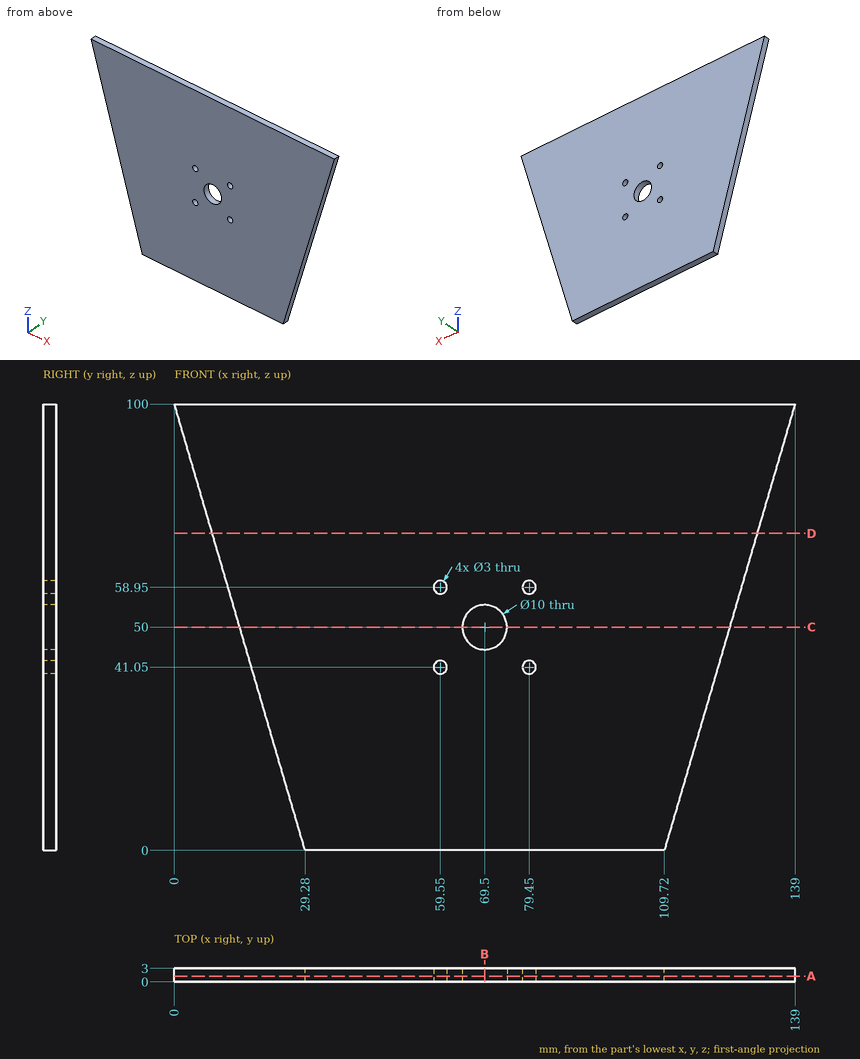
Geometry check sheet. Reference: drawing and pictorial views, mm from the part's lowest x, y, z. Coordinates: 2 decimals unless noted, no trailing zeros. Order: outer loops, then holes, each group sorted by start corner. A loop starts at its lowest first (then second) coordinate and runs counter-clockwise, first axis right, second up. Notation, with made-up numbers: (-35.75, -33) -> (-5.75, -33) arc R35 ccw to (-5.75, 1) -> close; hole circle Ø11 at (61.5, 4.25). An arc over 180 degrees is marked (long way). Put each result on its own line as item: value. Start each with the question number.
1) Cross-section at C-C (z = 50). Enter the section's corners in (x, y), plus the area to 3 significant figures.
2) Cross-section at B-B (x = 69.5). Enter the section's corners in (y, z), plus the area to 3 significant figures.
3) Cross-section at A-A (y = 1.3). Enter the section's corners in (x, z), plus the area to 3 significant figures.
4) Material ranges on L1, parallel to Z at x = 59.55, y = 1.95; L2, parallel to Z at x = 69.5, y = 2.2; L3, parallel to X at y = 1.55, z = 41.05, recorded low to high.
5) Go/stop test with a flat-tipped pin: pin 1 (1 mm diameter, centred on y = 2.5, z = 30, fed in from +X). Record where the tip stops, or that it passes through.
6) Cross-section at D-D (z = 71). Enter the section's corners in (x, y), plus the area to 3 significant figures.
Geometry check:
1. outline: (14.64, 0) -> (64.5, 0) -> (64.5, 3) -> (14.64, 3) -> close; (74.5, 0) -> (124.36, 0) -> (124.36, 3) -> (74.5, 3) -> close
1. area: 299 mm^2
2. outline: (0, 0) -> (3, 0) -> (3, 45) -> (0, 45) -> close; (0, 55) -> (3, 55) -> (3, 100) -> (0, 100) -> close
2. area: 270 mm^2
3. outline: (0, 100) -> (29.28, 0) -> (109.72, 0) -> (139, 100) -> close; hole circle Ø3 at (59.55, 41.05); hole circle Ø3 at (59.55, 58.95); hole circle Ø10 at (69.5, 50); hole circle Ø3 at (79.45, 41.05); hole circle Ø3 at (79.45, 58.95)
3. area: 10,900 mm^2
4. L1: z = 0 to 39.55, 42.55 to 57.45, 60.45 to 100
4. L2: z = 0 to 45, 55 to 100
4. L3: x = 17.26 to 58.05, 61.05 to 77.95, 80.95 to 121.74
5. pin 1: stops at x = 118.65
6. outline: (8.49, 0) -> (130.51, 0) -> (130.51, 3) -> (8.49, 3) -> close
6. area: 366 mm^2
